Check sheet for the modelled part. Datum: model origin and axes. Units: mm. Round coordinates to 2 decimals unless told otherwise and drop trailing zeros. Write each loop counter-clockwise with the first axis right and the second up, starting at its lowest first coordinate (ties: lowest second). Pieces come first, ordered by that corner, then holes.
Item 1: Cross-section at B-B on x = 1.8. Count the separate pieces of the cut face and the enclosed holes in it, plus the area to 3 significant figures.
Item 2: Material ranges on line 1 (Y direction, x = 1.5, z = 23); line 2 (Z direction, x = 2.9, y = -67.5); line 3 (Y direction, x = 2.2, z = 11), recorded low to high.
Item 3: Go/stop test with a flat-tipped pin: pin 1 Ø10 at (y, z) = (-6.5, 12) entering from +X. Record where the tip stops, or that it passes through.
Item 4: Cross-section at A-A on y = -71. Enter the section's corners in (x, z), plus the area to 3 significant figures.
Item 5: Cross-section at D-D on y = 2. Enter the section's corners in (x, z).
Item 6: Cross-section at C-C on z = 23. Enter the section's corners in (x, y).
from build123d import *

# Parameters (mm, degrees)
SKETCH_W        = 185
SKETCH_H        = 52
PAD_DEPTH       = 3
SHAPEBINDER_R   = 11.8
SHAPEBINDER_R_2 = 1.55
SHAPEBINDER_W   = 12.9
SHAPEBINDER_H   = 19.4
SHAPEBINDER_R_3 = 1.6
POCKET_DEPTH    = 5


with BuildPart() as part:
    # Sketch → Pad (new body)
    with BuildSketch(Plane.YZ):
        with Locations((0, 23)):
            Rectangle(SKETCH_W, SKETCH_H)
    extrude(amount=PAD_DEPTH)

    # ShapeBinder → Pocket (cut)
    with BuildSketch(Plane(origin=(0, 0.410224, 23), x_dir=(0, -1, 0), z_dir=(1, 0, 0))):
        with Locations((-67.839494, 0)):
            Circle(SHAPEBINDER_R)
        with Locations((-58.339494, -12)):
            Circle(SHAPEBINDER_R_2)
        with Locations((-77.339494, 12)):
            Circle(SHAPEBINDER_R_2)
        with BuildLine():
            ThreePointArc((-24.986195, 14.35), (-39.336195, 0), (-24.986195, -14.35))
            Line((-24.986195, -14.35), (0.713805, -14.35))
            ThreePointArc((0.713805, -14.35), (15.063805, 0), (0.713805, 14.35))
            Line((0.713805, 14.35), (-24.986195, 14.35))
        make_face()
        with Locations((41.785392, 0)):
            Circle(SHAPEBINDER_R)
        with Locations((32.285392, 12)):
            Circle(SHAPEBINDER_R_2)
        with Locations((51.285392, -12)):
            Circle(SHAPEBINDER_R_2)
        with Locations((73.189494, 0)):
            Rectangle(SHAPEBINDER_W, SHAPEBINDER_H)
        with Locations((12.863805, -12.2)):
            Circle(SHAPEBINDER_R_3)
        with Locations((12.863805, 12.2)):
            Circle(SHAPEBINDER_R_3)
        with Locations((-37.136195, 12.2)):
            Circle(SHAPEBINDER_R_3)
        with Locations((-37.136195, -12.2)):
            Circle(SHAPEBINDER_R_3)
    extrude(amount=POCKET_DEPTH, mode=Mode.SUBTRACT)


solid = part.part
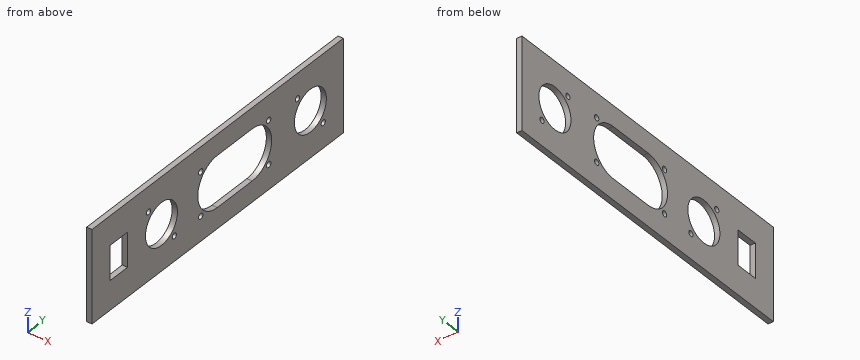
Response values:
1. separate pieces: 1
1. enclosed holes: 12
1. area: 7,050 mm2
2. line 1: y = -92.5 to -79.23, -66.33 to -53.18, -29.58 to -14.65, 39.75 to 56.45, 80.05 to 92.5
2. line 2: z = -3 to 13.3, 32.7 to 49
2. line 3: y = -92.5 to -33.43, -30.33 to -14.04, -10.87 to -8.17, 33.27 to 35.96, 39.13 to 76.2, 79.3 to 92.5
3. pin 1: stops at x = 3
4. outline: (0, -3) - (3, -3) - (3, 13.3) - (0, 13.3) - close; (0, 32.7) - (3, 32.7) - (3, 49) - (0, 49) - close
4. area: 97.8 mm2
5. outline: (0, -3) - (3, -3) - (3, 8.65) - (0, 8.65) - close; (0, 37.35) - (3, 37.35) - (3, 49) - (0, 49) - close
6. outline: (0, -92.5) - (3, -92.5) - (3, -79.23) - (0, -79.23) - close; (0, -66.33) - (3, -66.33) - (3, -53.18) - (0, -53.18) - close; (0, -29.58) - (3, -29.58) - (3, -14.65) - (0, -14.65) - close; (0, 39.75) - (3, 39.75) - (3, 56.45) - (0, 56.45) - close; (0, 80.05) - (3, 80.05) - (3, 92.5) - (0, 92.5) - close
